Job drawing, mm, ordinate dimensions from the low corner. One solid piece. A direction names the side the tool comes from. Round coordinates to 2 decimals unless told otherwise and drop trailing zeros. Write each loop counter-clockwise with the first axis right and the second up, starting at its lowest first coordinate (ties: lowest second). Pieces come first, ordered by that corner, then holes.
1) Saw through at C-C (z = 3). Write the cut outline in (x, y), plus the area to 3 significant figures.
2) Pull direction X, two halves, no side cores. Call the marked faces 1 and 2: +X half, -X half, draft (parallel to the pull), parting line (faces both ways), or undercut.
3) Saw through at A-A (y = 2.5). State how many separate pieces and enclosed holes the cut face has, plus the area to 3 significant figures.
4) Saw through at D-D (y = 5.65). Write the cut outline in (x, z), plus the area to 3 significant figures.
5) Wall check: probe 1 along X at (y, z) = (2.5, 7.25); probe 2 along X at (y, z) = (4.95, 7.25); probe 3 along Z at (x, y) = (3.5, 3.4). Give the ranges that are in metal, low to high.
6) Which spindle directions (+Z, -Z, +X, -X, +Y, -Y) get a long thin tool onto all of the face, cutting with end or side? Do the marked faces 3, 4, 5, 6 and 7. Say none if no direction does.
7) Flat gauge pins, fed straight in: pin 1 (1.9 mm diameter, centred on x = 5, y = 2.5, fed in from -Z); pin 2 (0.8 mm diameter, centred on y = 4.5, z = 6.5, fed in from +X); pin 3 (1 mm diameter, centred on y = 2.5, z = 2.5, fed in from -X). Where does each tip first touch, or does it go through?
8) Saw through at B-B (x = 28.5). Write the cut outline in (y, z), plus the area to 3 significant figures.
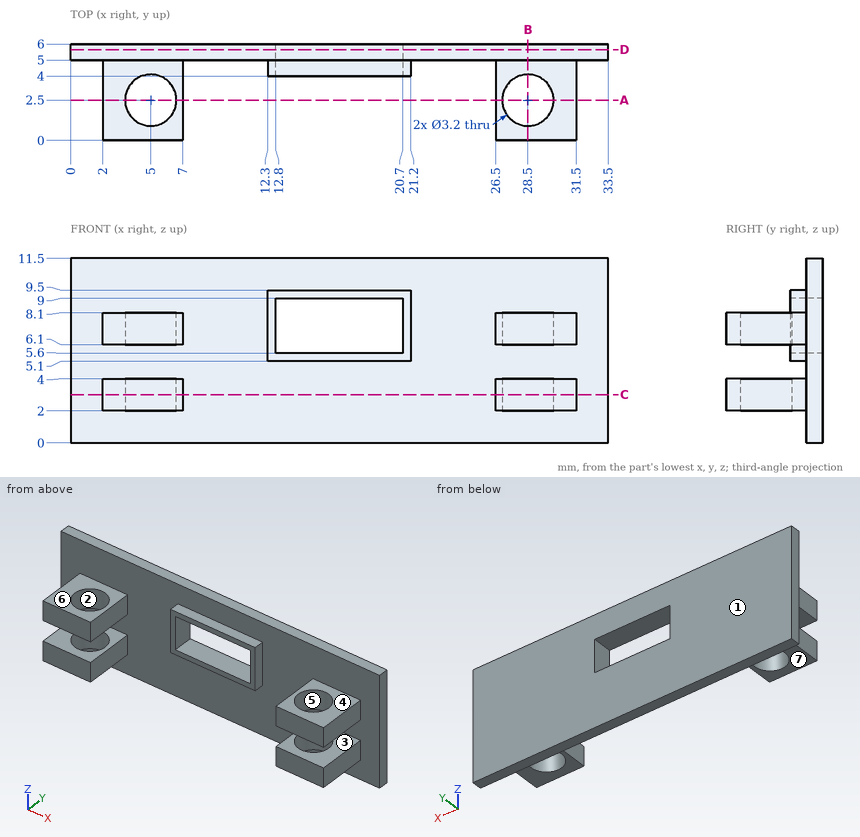
Evaluation:
1. outline: (0, 5) - (2, 5) - (2, 0) - (7, 0) - (7, 5) - (26.5, 5) - (26.5, 0) - (31.5, 0) - (31.5, 5) - (33.5, 5) - (33.5, 6) - (0, 6) - close; hole circle Ø3.2 at (5, 2.5); hole circle Ø3.2 at (28.5, 2.5)
1. area: 67.4 mm2
2. face 1: draft
2. face 2: undercut
3. separate pieces: 8
3. enclosed holes: 0
3. area: 14.4 mm2
4. outline: (0, 0) - (33.5, 0) - (33.5, 11.5) - (0, 11.5) - close; hole (12.8, 5.6) - (20.7, 5.6) - (20.7, 9) - (12.8, 9) - close
4. area: 358 mm2
5. probe 1: x = 2 to 3.4, 6.6 to 7, 26.5 to 26.9, 30.1 to 31.5
5. probe 2: x = 2 to 7, 12.3 to 12.8, 20.7 to 21.2, 26.5 to 31.5
5. probe 3: z = 2 to 4, 6.1 to 8.1
6. face 3: +X, -X, -Y
6. face 4: +Z, +X, -Y
6. face 5: +Z, -Z
6. face 6: +Z, -X, -Y
6. face 7: -Z, +X, -X, -Y
7. pin 1: passes through
7. pin 2: stops at x = 31.5
7. pin 3: stops at x = 2
8. outline: (0, 2) - (0.9, 2) - (0.9, 4) - (0, 4) - close; (0, 6.1) - (0.9, 6.1) - (0.9, 8.1) - (0, 8.1) - close; (4.1, 2) - (5, 2) - (5, 0) - (6, 0) - (6, 11.5) - (5, 11.5) - (5, 8.1) - (4.1, 8.1) - (4.1, 6.1) - (5, 6.1) - (5, 4) - (4.1, 4) - close
8. area: 18.7 mm2
